Here's how the part is built. I have some questions about the finished solid (model axes, mm). Give positions to 0.01 mm unless a question says otherwise; leave off trailing zeros. Write each loop counter-clockwise with the first axis right and the second up, starting at its lowest first coordinate (ties: lowest second). Pieces come first, ordered by that corner, then holes. Notation, with made-up numbers: (47.5, 18) -> (77.5, 18) arc R14 cw to (77.5, 38) -> close; hole circle Ø5 at (83, 39). An arc over 180 degrees is marked (long way). Put each result on its own line as item: value. Start each with the question number.
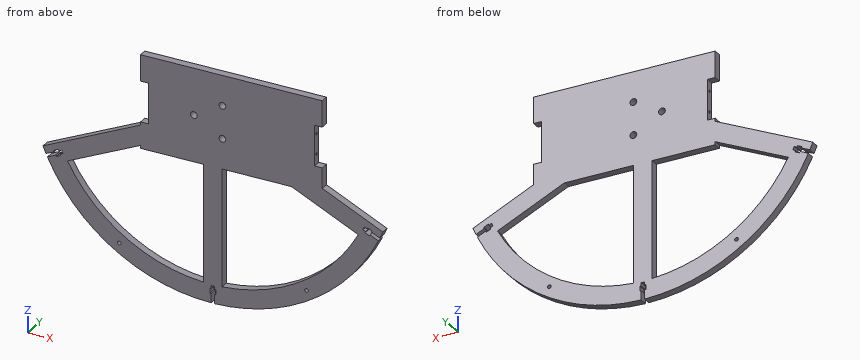
from build123d import *

# Parameters (mm, degrees)
BOSS_EXTRUDE1_DEPTH               = 3.175
SKETCH2_W                         = 2.75
SKETCH2_H                         = 2.5
SKETCH2_H_2                       = 4
SKETCH2_W_2                       = 1.125
SKETCH2_H_3                       = 7.5
CUT_EXTRUDE1_DEPTH                = 204.460831631
CIRPATTERN1_COUNT                 = 2
CIRPATTERN1_ANGLE                 = 65
CIRPATTERN1_THE_OTHER_WAY_COUNT   = 2
CIRPATTERN1_THE_OTHER_WAY_ANGLE   = 65
F_3_0_3_DIAMETER_HOLE1_D          = 3
M5_CLEARANCE_HOLE1_D              = 5.5
SKETCH9_W                         = 6.35
SKETCH9_H                         = 33.16
CUT_EXTRUDE2_DEPTH                = 204.530492207
M2_5X0_45_TAPPED_HOLE1_AT_2_COUNT = 2
M2_5X0_45_TAPPED_HOLE1_AT_2_PITCH = 16.83


with BuildPart() as part:
    # Sketch1 → Boss-Extrude1 (new, symmetric)
    with BuildSketch(Plane(origin=(0, 0, 0), x_dir=(1, 0, 0), z_dir=(0, 1, 0))):
        with BuildLine():
            Line((88.95, 33.202731801), (138.254290129, 56.193699868))
            ThreePointArc((138.254290129, 56.193699868), (0, 149.238), (-138.254290129, 56.193699868))
            Line((-138.254290129, 56.193699868), (-58.85, 19.16687129))
            Line((-58.85, 19.16687129), (-58.85, -38.1))
            Line((-58.85, -38.1), (88.95, -38.1))
            Line((88.95, -38.1), (88.95, 33.202731801))
        make_face()
        with BuildLine():
            Line((-7.5, 11.821590418), (-7.5, 11.772641828))
            Line((-7.5, 11.772641828), (-7.544362488, 11.793328396))
            ThreePointArc((-7.544362488, 11.793328396), (-7.522194517, 11.807480241), (-7.5, 11.821590418))
        make_face(mode=Mode.SUBTRACT)
        with BuildLine():
            ThreePointArc((7.5, 11.821590418), (7.522194517, 11.807480241), (7.544362488, 11.793328396))
            Line((7.544362488, 11.793328396), (7.5, 11.772641828))
            Line((7.5, 11.772641828), (7.5, 11.821590418))
        make_face(mode=Mode.SUBTRACT)
        with BuildLine():
            Line((-7.5, 134.028320306), (-7.5, 38.1))
            Line((-7.5, 38.1), (-58.85, 38.1))
            Line((-58.85, 38.1), (-58.85, 35.717540075))
            Line((-58.85, 35.717540075), (-118.301273414, 63.440124154))
            ThreePointArc((-118.301273414, 63.440124154), (-72.126024825, 113.215180903), (-7.5, 134.028320306))
        make_face(mode=Mode.SUBTRACT)
        with BuildLine():
            ThreePointArc((7.5, 134.028320306), (72.126024825, 113.215180903), (118.301273414, 63.440124154))
            Line((118.301273414, 63.440124154), (63.959201798, 38.1))
            Line((63.959201798, 38.1), (7.5, 38.1))
            Line((7.5, 38.1), (7.5, 134.028320306))
        make_face(mode=Mode.SUBTRACT)
    extrude(amount=BOSS_EXTRUDE1_DEPTH, both=True)

    # Sketch2 → Cut-Extrude1 (cut, symmetric)
    with BuildSketch(Plane(origin=(0, 0, 0), x_dir=(1, 0, 0), z_dir=(0, 1, 0))):
        with Locations((0, 136.488)):
            Rectangle(SKETCH2_W, SKETCH2_H)
        with Locations((0, 139.738)):
            Rectangle(SKETCH2_W, SKETCH2_H_2)
        with Locations((1.9375, 139.738)):
            Rectangle(SKETCH2_W_2, SKETCH2_H_2)
        with Locations((0, 145.488)):
            Rectangle(SKETCH2_W, SKETCH2_H_3)
        with Locations((-1.9375, 139.738)):
            Rectangle(SKETCH2_W_2, SKETCH2_H_2)
    cut_extrude1 = extrude(amount=CUT_EXTRUDE1_DEPTH, both=True, mode=Mode.SUBTRACT)

    # CirPattern1: Cut-Extrude1 ×2 about axis
    cirpattern1_axis = Axis((0, 0, 0), (0, 1, 0))
    for i in range(1, CIRPATTERN1_COUNT):
        add(cut_extrude1.rotate(cirpattern1_axis, i * CIRPATTERN1_ANGLE / (CIRPATTERN1_COUNT - 1)), mode=Mode.SUBTRACT)

    # CirPattern1 the other way: Cut-Extrude1 ×2 about axis
    cirpattern1_the_other_way_axis = Axis((0, 0, 0), (0, -1, 0))
    for i in range(1, CIRPATTERN1_THE_OTHER_WAY_COUNT):
        add(cut_extrude1.rotate(cirpattern1_the_other_way_axis, i * CIRPATTERN1_THE_OTHER_WAY_ANGLE / (CIRPATTERN1_THE_OTHER_WAY_COUNT - 1)), mode=Mode.SUBTRACT)

    # Ø3.0 (3) Diameter Hole1 (through all)
    with Locations(Plane(origin=(0, 3.175, 0), x_dir=(1, 0, 0), z_dir=(0, 1, 0))):
        with Locations((76.155771888, 119.540616747), (-76.155771888, 119.540616747)):
            Hole(F_3_0_3_DIAMETER_HOLE1_D / 2)

    # M5 Clearance Hole1 (through all)
    with Locations(Plane(origin=(0, 3.175, 0), x_dir=(1, 0, 0), z_dir=(0, 1, 0))):
        with Locations((-15.5, 0), (7.75, 13.423393759), (7.75, -13.423393759)):
            Hole(M5_CLEARANCE_HOLE1_D / 2)

    # Sketch9 → Cut-Extrude2 (cut, through all)
    with BuildSketch(Plane(origin=(0, 3.175, 0), x_dir=(1, 0, 0), z_dir=(0, 1, 0))):
        with Locations((-55.675, 0)):
            Rectangle(SKETCH9_W, SKETCH9_H)
        with Locations((85.775, 0)):
            Rectangle(SKETCH9_W, SKETCH9_H)
    extrude(amount=-CUT_EXTRUDE2_DEPTH, mode=Mode.SUBTRACT)

    # Sketch11 → M2.5x0.45 Tapped Hole1 (revolve, cut)
    with BuildSketch(Plane(origin=(-52.5, 0, -8.415), x_dir=(0, 0, 1), z_dir=(0, 1, 0))):
        Polygon((0, 0), (0, 6.965882135), (1.025, 6.35), (1.025, 0), align=None)
    m2_5x0_45_tapped_hole1 = revolve(axis=Axis((-58.85, 0, -8.415), (1, 0, 0)), mode=Mode.SUBTRACT)

    # M2.5x0.45 Tapped Hole1 at 2: M2.5x0.45 Tapped Hole1 ×2
    with Locations(*[(0, 0, i * M2_5X0_45_TAPPED_HOLE1_AT_2_PITCH) for i in range(1, M2_5X0_45_TAPPED_HOLE1_AT_2_COUNT)]):
        add(m2_5x0_45_tapped_hole1, mode=Mode.SUBTRACT)

    # Mirror1: M2.5x0.45 Tapped Hole1 across plane
    add(m2_5x0_45_tapped_hole1.mirror(Plane.ZY.offset(-15.05)), mode=Mode.SUBTRACT)

    # Mirror1 copy 1 sketch → Mirror1 copy 1 (revolve, cut)
    with BuildSketch(Plane(origin=(82.6, 0, 8.415), x_dir=(0, 0, 1), z_dir=(0, 1, 0))):
        Polygon((0, 0), (0, -6.965882135), (1.025, -6.35), (1.025, 0), align=None)
    revolve(axis=Axis((88.95, 0, 8.415), (1, 0, 0)), mode=Mode.SUBTRACT)


solid = part.part
1) I need wall thicknesses on probe 1 along X at (y, z) = (2.25, -82); probe 2 along Z at (x, y) = (7.75, -0.75); probe 3 along X at (y, z) = (-0.5, -67). Which ranges of each line are inside material? Lowest first, please.
2) I want a section at D-D, the plane x = 51.5. Write out the boundary of the cut face in (y, z) (3 decimals), and give its area (3 significant figures).
3) I want a section at C-C, the plane x = -15.5. Write out the boundary of the cut face in (y, z) (3 decimals).
4) I want a section at B-B, the plane z = -126. Write out the boundary of the cut face in (x, y) (3 decimals), and give its area (3 significant figures).
5) I want a section at A-A, the plane x = 14.5. Write out the boundary of the cut face in (y, z) (3 decimals), and give its area (3 significant figures).
6) I'm going to push flat-ended pins straight in: pin 1 Ø1.2 at (y, z) = (0, -8.415) entering from +X; pin 2 Ø1 at (y, z) = (-0.5, -91) entering from -X; pin 3 Ø2 at (x, y) = (0, 0.5) entering from -Z. Where does each tip first touch, or does it pass through?
Established:
1. probe 1: x = -124.69 to -106.28, -7.5 to 7.5, 106.28 to 124.69
1. probe 2: z = -149.04 to -134.01, -38.1 to -16.17, -10.67 to 10.67, 16.17 to 38.1
1. probe 3: x = -133.35 to -116.32, -7.5 to 7.5, 116.32 to 133.35
2. outline: (-3.175, -140.07) -> (3.175, -140.07) -> (3.175, -123.966) -> (-3.175, -123.966) -> close; (-3.175, -38.1) -> (3.175, -38.1) -> (3.175, 38.1) -> (-3.175, 38.1) -> close
2. area: 586 mm2
3. outline: (-3.175, -148.431) -> (3.175, -148.431) -> (3.175, -133.34) -> (-3.175, -133.34) -> close; (-3.175, -38.1) -> (3.175, -38.1) -> (3.175, -2.75) -> (-3.175, -2.75) -> close; (-3.175, 2.75) -> (3.175, 2.75) -> (3.175, 38.1) -> (-3.175, 38.1) -> close
4. outline: (-79.975, -3.175) -> (-46.302, -3.175) -> (-46.302, 3.175) -> (-79.975, 3.175) -> close; (-7.5, -3.175) -> (7.5, -3.175) -> (7.5, 3.175) -> (-7.5, 3.175) -> close; (46.302, -3.175) -> (79.975, -3.175) -> (79.975, 3.175) -> (46.302, 3.175) -> close
4. area: 523 mm2
5. outline: (-3.175, -148.532) -> (3.175, -148.532) -> (3.175, -133.453) -> (-3.175, -133.453) -> close; (-3.175, -38.1) -> (3.175, -38.1) -> (3.175, 38.1) -> (-3.175, 38.1) -> close
5. area: 580 mm2
6. pin 1: stops at x = 75.99
6. pin 2: stops at x = -118.67
6. pin 3: stops at z = -135.24
